Can you work these out from the model? Positions are in its coordinate system, mm. A direction names the side the tool comes from. Round coordinates to 2 decimals unless told otherwise and drop trailing zeros. Loops run counter-clockwise (first coordinate to the right, second up) from the corner with the lowest first, then second, coordinate; pieces in that order, holes last.
from build123d import *

# Parameters (mm, degrees)
SKETCH1_W           = 38.1
SKETCH1_H           = 25.4
SKETCH1_R           = 1.8288
SKETCH1_W_2         = 6.35
SKETCH1_H_2         = 12.7
BOSS_EXTRUDE1_DEPTH = 6.35


with BuildPart() as part:
    # Sketch1 → Boss-Extrude1 (new body)
    # profile 1 of 3: a face of its own
    with BuildSketch(Plane(origin=(0, 0, 0), x_dir=(1, 0, 0), z_dir=(0, 1, 0))):
        with Locations((19.05, -12.7)):
            Rectangle(SKETCH1_W, SKETCH1_H)
        with Locations(Location((19.05, -12.7, 0), (0, 0, 270))):
            Circle(SKETCH1_R, mode=Mode.SUBTRACT)
    # profile 2 of 3: a face of its own
    with BuildSketch(Plane(origin=(0, 0, 0), x_dir=(1, 0, 0), z_dir=(0, 1, 0))):
        with Locations((41.275, -12.7)):
            Rectangle(SKETCH1_W_2, SKETCH1_H_2)
    # profile 3 of 3: a face of its own
    with BuildSketch(Plane(origin=(0, 0, 0), x_dir=(1, 0, 0), z_dir=(0, 1, 0))):
        with Locations((-3.175, -12.7)):
            Rectangle(SKETCH1_W_2, SKETCH1_H_2)
    extrude(amount=BOSS_EXTRUDE1_DEPTH)


solid = part.part
(1) If we section it at C-C, the plane y = 1.5: List the corners of the cut face in (x, z) for me.
Worked answers:
outline: (-6.35, 6.35) - (0, 6.35) - (0, 0) - (38.1, 0) - (38.1, 6.35) - (44.45, 6.35) - (44.45, 19.05) - (38.1, 19.05) - (38.1, 25.4) - (0, 25.4) - (0, 19.05) - (-6.35, 19.05) - close; hole circle Ø3.66 at (19.05, 12.7)
(2) If we mould it in two halves opening along Z, with no side actions, what happens to faces 1 (the cylindrical face through (20.863, 3.131, 12.462)), 2 (the flat face through (-3, 3, 19.05)), 3 (the flat face through (0, 3, 22))? For each: released by +Z, released by -Z, zero draft, split by the parting line, or undercut.
Worked answers:
face 1: undercut
face 2: released by +Z
face 3: zero draft
(3) Will this pin go through, and if not, where does the flat tip stop? P1, Ø3, axis at x = -4.5, y = 3.5, coming from the +Z side.
Worked answers:
P1: stops at z = 19.05
(4) For faces 4 (the flat face through (38.1, 3, 3)), 5 (the flat face through (41, 3, 19.05)), 6 (the flat face through (-3, 3, 6.35)), 7 (the flat face through (-6.35, 3, 13)), which set-ups out of +Z, -Z, +X, -X, +Y, -Y let a thin tool reach every point of the face, with its end or its side?
Worked answers:
face 4: -Z, +X, +Y, -Y
face 5: +Z, +X, +Y, -Y
face 6: -Z, -X, +Y, -Y
face 7: +Z, -Z, -X, +Y, -Y
(5) If we section it at D-D, the plane z = 21.75: List the corners of the cut face in (x, y) for me.
Worked answers:
outline: (0, 0) - (38.1, 0) - (38.1, 6.35) - (0, 6.35) - close
(6) If we section it at B-B, the plane x = 19.05: List the corners of the cut face in (y, z) for me.
Worked answers:
outline: (0, 0) - (6.35, 0) - (6.35, 10.87) - (0, 10.87) - close; (0, 14.53) - (6.35, 14.53) - (6.35, 25.4) - (0, 25.4) - close
(7) If I drill on line 1 (X direction, y = 1.5, z = 12.7); line 2 (X direction, y = 1.25, z = 23.25); line 3 (X direction, y = 5.25, z = 11.5), over which ranges is the centre line in solid material (lowest first)?
Worked answers:
line 1: x = -6.35 to 17.22, 20.88 to 44.45
line 2: x = 0 to 38.1
line 3: x = -6.35 to 17.67, 20.43 to 44.45
(8) If we section it at A-A, the plane z = 12.7: List the corners of the cut face in (x, y) for me.
Worked answers:
outline: (-6.35, 0) - (17.22, 0) - (17.22, 6.35) - (-6.35, 6.35) - close; (20.88, 0) - (44.45, 0) - (44.45, 6.35) - (20.88, 6.35) - close
